Read the model definition and answer for the solid it produces. Units are mm, in the model's axes. Face numbers are marked on the shaded views. A direction names the side the tool comes from. Give positions to 0.01 mm unless a question says otherwise; leave off trailing zeros. Write each loop counter-clockwise with the first axis right and the second up, starting at its lowest first coordinate (ties: lowest second). Pieces come first, ordered by that corner, then holes. Notation, with made-up numbers: (-32.5, 53) -> (4.5, 53) arc R28 ccw to (4.5, 72) -> close; hole circle Ø5 at (2.25, 36). An arc over 180 degrees is marked (long way). Answer as CSV lines item,"result". Start each with the question number.
1. The part is cut by section D-D, the plane x = -39.5. Determine the outline of the cut face in (y, z), and give its area (3 significant figures).
2. For a pull along X with two mould halves and no side action, classify the marked faces 3, 4 and 5 as pulls with the +X half, pulls with the -X half, needs draft (parallel to the pull), parting line crosses it, or undercut.
3. Find the intervals of material crossed by line 1 (X direction, y = 0.5, z = 3.75); line 2 (Z direction, x = -44, y = 6.5); line 3 (Y direction, x = -24, z = 3.5), in increasing order.
4. The part is cut by section B-B, the plane z = 4. Determine the outline of the cut face in (x, y), and give its area (3 significant figures).
5. The part is cut by section A-A, the plane y = -3. Determine the outline of the cut face in (x, z).
6. Given pin 1 (2 mm diameter, centred on y = -5, z = 5, fed in from -X); pin 2 (2 mm diameter, centred on x = -43, z = 2.5, fed in from -Y); pin 3 (4 mm diameter, centred on y = -4, z = 4, fed in from -X), each flat-ended and moving along its own axis, determine where each tip first touches the part or whether it passes through.
7. The part is cut by section C-C, the plane x = 44. Determine the outline of the cut face in (y, z).
8. A tool of negligible diameter and unlimited length cuts with its end or side. For the marked faces 1 and 2, from which of +Z, -Z, +X, -X, +Y, -Y can it reach the whole face along a straight path? Write none if from no direction.
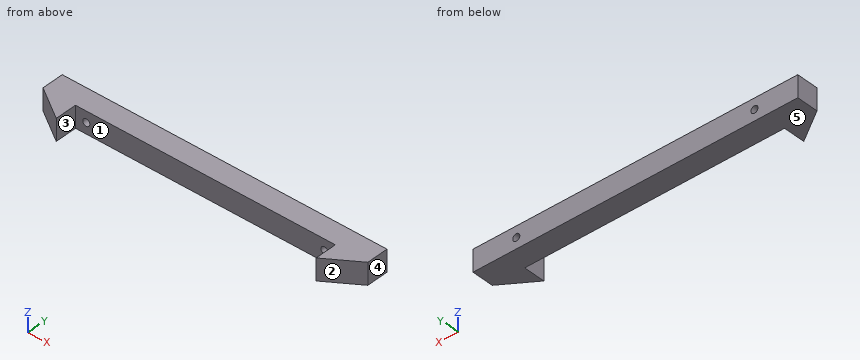
from build123d import *

# Parameters (mm, degrees)
BOSS_EXTRUDE1_DEPTH = 8
CUT_EXTRUDE1_REACH  = 63.057
SKETCH2_R           = 1.3


with BuildPart() as part:
    # Sketch1 → Boss-Extrude1 (new body)
    with BuildSketch(Plane(origin=(0, 0, 0), x_dir=(0, 1, 0), z_dir=(0, 0, 1))):
        Polygon((0, 48), (0, -48), (-8, -48), (0, -60), (8, -60), (8, 60), (0, 60), (-8, 48), align=None)
    extrude(amount=BOSS_EXTRUDE1_DEPTH)

    # Sketch2 → Cut-Extrude1 (cut, up to next)
    with BuildSketch(Plane.XZ, mode=Mode.PRIVATE) as cut_extrude1_sk1:
        with Locations((-44, 4)):
            Circle(SKETCH2_R)
    cut_extrude1_tool1 = extrude(cut_extrude1_sk1.sketch, amount=-CUT_EXTRUDE1_REACH, mode=Mode.PRIVATE) & part.part
    # Sketch2 → Cut-Extrude1 (cut, up to next)
    with BuildSketch(Plane.XZ, mode=Mode.PRIVATE) as cut_extrude1_sk2:
        with Locations(Location((44, 4, 0), (0, 0, 270))):
            Circle(SKETCH2_R)
    cut_extrude1_tool2 = extrude(cut_extrude1_sk2.sketch, amount=-CUT_EXTRUDE1_REACH, mode=Mode.PRIVATE) & part.part
    add(cut_extrude1_tool1.solids().sort_by_distance((-44, 0, 4))[0], mode=Mode.SUBTRACT)
    add(cut_extrude1_tool2.solids().sort_by_distance((44, 0, 4))[0], mode=Mode.SUBTRACT)


solid = part.part
Results found:
1,outline,"(0, 0) -> (8, 0) -> (8, 8) -> (0, 8) -> close"
1,area,"64.0 mm²"
2,face 3,"undercut"
2,face 4,"pulls with the +X half"
2,face 5,"needs draft"
3,line 1,"x = -60 to -45.28, -42.72 to 42.72, 45.28 to 60"
3,line 2,"z = 0 to 2.7, 5.3 to 8"
3,line 3,"y = 0 to 8"
4,outline,"(-60, 0) -> (-48, -8) -> (-48, 0) -> (-45.3, 0) -> (-45.3, 8) -> (-60, 8) -> close; (-42.7, 0) -> (42.7, 0) -> (42.7, 8) -> (-42.7, 8) -> close; (45.3, 0) -> (48, 0) -> (48, -8) -> (60, 0) -> (60, 8) -> (45.3, 8) -> close"
4,area,"1,010 mm²"
5,outline,"(-55.5, 0) -> (-48, 0) -> (-48, 8) -> (-55.5, 8) -> close; (48, 0) -> (55.5, 0) -> (55.5, 8) -> (48, 8) -> close"
6,pin 1,"stops at x = -54"
6,pin 2,"stops at y = 0"
6,pin 3,"stops at x = -57"
7,outline,"(0, 0) -> (8, 0) -> (8, 2.7) -> (0, 2.7) -> close; (0, 5.3) -> (8, 5.3) -> (8, 8) -> (0, 8) -> close"
8,face 1,"+Z, -Z, -Y"
8,face 2,"+Z, -Z, +X, -Y"
